Verification items for the finished model (mm, model axes). Face numbers are marked on the shaded views. A direction names the side the tool comes from. Give positions to 0.01 mm unless a question says otherwise; leave off trailing zeros. Write each loop counter-clockwise with the first axis right and the second up, starting at its lowest first coordinate (ties: lowest second). Pieces come first, ordered by that corner, then holes. Notation, with made-up numbers: M 7.5,25 L 26.5,25 A18 cw 26.5,30 Z; hole C 0,-38.75 d4. An arc over 180 degrees is marked long. Write item = value, one per line.
from build123d import *

# Parameters (mm, degrees)
EXTRUDE_1_DEPTH     = 16
SKETCH_1_3_R        = 9
EXTRUDE_2_DEPTH     = 25
EXTRUDE_3_DEPTH     = 25
CUT_EXTRUDE_1_DEPTH = 25


with BuildPart() as part:
    # Sketch 1 → Extrude 1 (new body)
    with BuildSketch(Plane.XY):
        with BuildLine():
            Line((-35, -50), (35, -50))
            ThreePointArc((35, -50), (42.071067812, -47.071067812), (45, -40))
            Line((45, -40), (45, 46.958512764))
            ThreePointArc((45, 46.958512764), (44.961331169, 48.481219091), (44.845424363, 50))
            Line((44.845424363, 50), (-44.845424363, 50))
            ThreePointArc((-44.845424363, 50), (-44.961331169, 48.481219091), (-45, 46.958512764))
            Line((-45, 46.958512764), (-45, -40))
            ThreePointArc((-45, -40), (-42.071067812, -47.071067812), (-35, -50))
        make_face()
        with BuildLine():
            Line((-44.845424363, 50), (44.845424363, 50))
            ThreePointArc((44.845424363, 50), (44.654940332, 51.495528733), (44.389564715, 52.979599532))
            Line((44.389564715, 52.979599532), (19.593043195, 174.014057595))
            ThreePointArc((19.593043195, 174.014057595), (19.898000702, 172.017317043), (20, 170))
            Line((20, 170), (20, 120))
            ThreePointArc((20, 120), (0, 100), (-20, 120))
            Line((-20, 120), (-20, 170))
            ThreePointArc((-20, 170), (-19.898000688, 172.017317185), (-19.593043138, 174.014057873))
            Line((-19.593043138, 174.014057873), (-44.389564715, 52.979599532))
            ThreePointArc((-44.389564715, 52.979599532), (-44.654940332, 51.495528733), (-44.845424363, 50))
        make_face()
    extrude(amount=EXTRUDE_1_DEPTH)

    # Sketch 1_3 → Extrude 2 (add)
    with BuildSketch(Plane.XY):
        with BuildLine():
            Line((-20, 170), (-20, 120))
            ThreePointArc((-20, 120), (0, 100), (20, 120))
            Line((20, 120), (20, 170))
            ThreePointArc((20, 170), (0, 190), (-20, 170))
        make_face()
        with Locations((0, 120)):
            Circle(SKETCH_1_3_R, mode=Mode.SUBTRACT)
        with Locations((0, 170)):
            Circle(SKETCH_1_3_R, mode=Mode.SUBTRACT)
    extrude(amount=EXTRUDE_2_DEPTH)

    # Sketch 2 → Extrude 3 (add)
    with BuildSketch(Plane.XY):
        with BuildLine():
            Line((18, -30), (-18, -30))
            ThreePointArc((-18, -30), (-26.485281374, -26.485281374), (-30, -18))
            Line((-30, -18), (-30, 18))
            ThreePointArc((-30, 18), (-26.485281374, 26.485281374), (-18, 30))
            Line((-18, 30), (18, 30))
            ThreePointArc((18, 30), (26.485281374, 26.485281374), (30, 18))
            Line((30, 18), (30, -18))
            ThreePointArc((30, -18), (26.485281374, -26.485281374), (18, -30))
        make_face()
    extrude(amount=EXTRUDE_3_DEPTH)

    # Sketch 3 → Cut-Extrude 1 (cut)
    with BuildSketch(Plane.XY.offset(25)):
        with BuildLine():
            Line((-4, 22), (-18, 22))
            ThreePointArc((-18, 22), (-20.828427125, 20.828427125), (-22, 18))
            Line((-22, 18), (-22, -18))
            ThreePointArc((-22, -18), (-20.828427125, -20.828427125), (-18, -22))
            Line((-18, -22), (-4, -22))
            Line((-4, -22), (-4, -18))
            Line((-4, -18), (4, -18))
            Line((4, -18), (4, -22))
            Line((4, -22), (18, -22))
            ThreePointArc((18, -22), (20.828427125, -20.828427125), (22, -18))
            Line((22, -18), (22, 18))
            ThreePointArc((22, 18), (20.828427125, 20.828427125), (18, 22))
            Line((18, 22), (4, 22))
            Line((4, 22), (4, 18))
            Line((4, 18), (-4, 18))
            Line((-4, 18), (-4, 22))
        make_face()
    extrude(amount=-CUT_EXTRUDE_1_DEPTH, mode=Mode.SUBTRACT)


solid = part.part
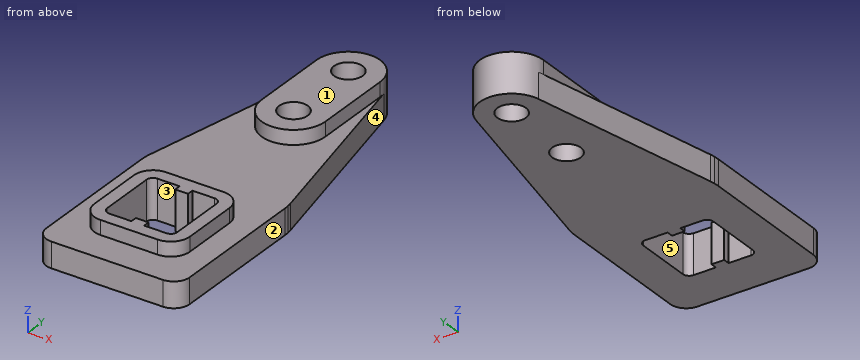
1) Cross-section at B-B on x = 0. Record the boundary of the cut face in (y, z).
From the geometry:
outline = M -50,0 L -18,0 L -18,25 L -30,25 L -30,16 L -50,16 Z; M 18,0 L 111,0 L 111,25 L 100,25 L 100,16 L 30,16 L 30,25 L 18,25 Z; M 129,0 L 161,0 L 161,25 L 129,25 Z; M 179,0 L 190,0 L 190,25 L 179,25 Z
2) Cross-section at D-D on z = 5.5. Record the boundary of the cut face in (x, y).
From the geometry:
outline = M -45,-40 A10 ccw -35,-50 L 35,-50 A10 ccw 45,-40 L 45,46.96 A30 ccw 44.39,52.98 L 19.59,174.01 A20 ccw -19.59,174.01 L -44.39,52.98 A30 ccw -45,46.96 Z; hole M -22,-18 A4 ccw -18,-22 L -4,-22 L -4,-18 L 4,-18 L 4,-22 L 18,-22 A4 ccw 22,-18 L 22,18 A4 ccw 18,22 L 4,22 L 4,18 L -4,18 L -4,22 L -18,22 A4 ccw -22,18 Z; hole C 0,120 d18; hole C 0,170 d18
3) Cross-section at C-C on y = 6. Record the boundary of the cut face in (x, z).
From the geometry:
outline = M -45,0 L -22,0 L -22,25 L -30,25 L -30,16 L -45,16 Z; M 22,0 L 45,0 L 45,16 L 30,16 L 30,25 L 22,25 Z
4) Depth check by flat-ended pin: P1, Ø4.5, axis at y = 135.5, z = 19.5, coming from the +X side; P2, Ø10, axis at y = 124.5, z = 3.5, coming from the +X side; P3, Ø4, axis at x = 20.5, y = 63, coming from the +Z side; P4, Ø2, axis at x = 16, y = 19.5, coming from the -Z side. Enter the tip coordinate at first touch or a pass-through.
From the geometry:
P1 = 20
P2 = 30.76
P3 = 16
P4 = through
5) Cross-section at A-A on z = 21.5. Count the separate pieces of the cut face and the enclosed holes in it, plus the area to 3 significant figures.
From the geometry:
separate_pieces = 2
enclosed_holes = 3
area = 4,370 mm^2
6) Material ranges on probe 1 along Y at (x, z) = (0, 17.25); probe 2 along Y at (x, z) = (0, 13); probe 3 along Y at (x, z) = (6, 19.5), recorded low to high. Write a range as from..to.
From the geometry:
probe_1 = -30..-18, 18..30, 100..111, 129..161, 179..190
probe_2 = -50..-18, 18..111, 129..161, 179..190
probe_3 = -30..-22, 22..30, 100.92..113.29, 126.71..163.29, 176.71..189.08
7) Draft check along X on the marked faces 1, 2 and 3. Enter one of: +X half, -X half, draft (parallel to the pull), parting line (faces both ways), or undercut.
From the geometry:
face_1 = draft
face_2 = +X half
face_3 = undercut
8) Tool access check on the marked faces 4 and 5. Record the directions out of +Z, -Z, +X, -X, +Y, -Y that give a thin tool (end or side, any length) a straight path to the whole face; none if there is none.
From the geometry:
face_4 = +Z, -Z, +X, +Y
face_5 = +Z, -Z
